Design review of the part shown in the three views and the two pictorial views. Dimensions are in mm from the part's minimum x, y and z. A direction names the side the tool comes from. Round coordinates to 2 decimals unless told otherwise and drop trailing zeros. Order: outer loops, then holes, each group sorted by start corner. A loop starts at its lowest first (then second) coordinate and runs counter-clockwise, first axis right, second up.
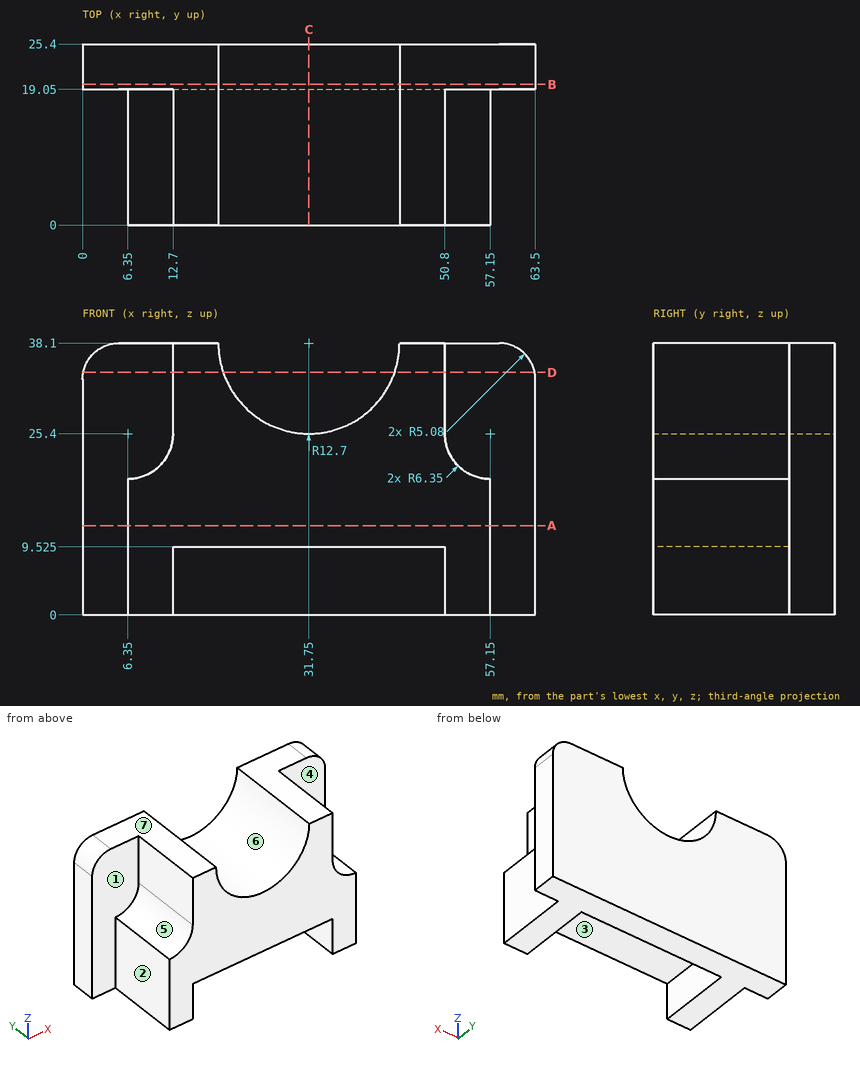
1) Take a section at D-D on z = 34. Give the boundary of the cut face in (x, y), plus the area to 3 significant figures.
Results:
outline: (0.1, 19.05) - (12.7, 19.05) - (12.7, 0) - (19.73, 0) - (19.73, 25.4) - (0.1, 25.4) - close; (43.77, 0) - (50.8, 0) - (50.8, 19.05) - (63.4, 19.05) - (63.4, 25.4) - (43.77, 25.4) - close
area: 517 mm2
2) The part is to be moulded in two halves that separate along X. For the marked faces 5, 6 and 7, say which applies: released by +X, released by -X, zero draft, split by the parting line, or undercut.
Results:
face 5: released by -X
face 6: undercut
face 7: zero draft
3) For the marked faces 1, 2, 3 and 4, list the 3-axis set-ups (+Z, -Z, +X, -X, +Y, -Y) from which the entire face can be reached by the end or side of a thin tool; tool diameter is ignored.
Results:
face 1: +Z, -X, -Y
face 2: +Z, -Z, -X, -Y
face 3: -Z, -Y
face 4: +Z, +X, -Y
4) To check wall thickness, follow line 1 along X through (y, z) = (6.25, 2.5); line 2 along X through (y, z) = (10.25, 17); line 3 along Y through (x, z) = (4.5, 31). State the ranges of each line that lie inside material, in increasing order.
Results:
line 1: x = 6.35 to 12.7, 50.8 to 57.15
line 2: x = 6.35 to 57.15
line 3: y = 19.05 to 25.4
5) Take a section at C-C on x = 31.75. Give the boundary of the cut face in (y, z) (3 decimals), plus the area to 3 significant figures.
Results:
outline: (0, 9.525) - (19.05, 9.525) - (19.05, 0) - (25.4, 0) - (25.4, 25.4) - (0, 25.4) - close
area: 464 mm2
6) Take a section at A-A on z = 12.5. Give the boundary of the cut face in (x, y), plus the area to 3 significant figures.
Results:
outline: (0, 19.05) - (6.35, 19.05) - (6.35, 0) - (57.15, 0) - (57.15, 19.05) - (63.5, 19.05) - (63.5, 25.4) - (0, 25.4) - close
area: 1,370 mm2
7) Take a section at B-B on y = 19.75. Give the boundary of the cut face in (x, z), plus the area to 3 significant figures.
Results:
outline: (0, 0) - (63.5, 0) - (63.5, 33.02) arc R5.08 ccw to (58.42, 38.1) - (44.45, 38.1) arc R12.7 cw to (19.05, 38.1) - (5.08, 38.1) arc R5.08 ccw to (0, 33.02) - close
area: 2,150 mm2
8) Clearance check with flat-ended pins moving along their axes: P1, Ø7.5, axis at x = 27, z = 6.5, coming from the -Y side; P2, Ø10, axis at y = 8, z = 31.5, coming from the +X side; P3, Ø1.5, axis at y = 3, z = 29.5, coming from the -X side; P4, Ø6, axis at x = 28.5, y = 18, coming from the +Z side. State where each tip first meets the part, or that it passes through.
Results:
P1: stops at y = 0
P2: stops at x = 50.8
P3: stops at x = 12.7
P4: stops at z = 27.04
